from build123d import *

# Parameters (mm, degrees)
SKETCH1_W           = 3.81
SKETCH1_H           = 13.335
SKETCH1_R           = 1.1049
BOSS_EXTRUDE1_DEPTH = 9.525
SKETCH2_W           = 2.54
SKETCH2_H           = 13.335
BOSS_EXTRUDE2_DEPTH = 9.525


with BuildPart() as part:
    # Sketch1 → Boss-Extrude1 (new body)
    with BuildSketch(Plane(origin=(0, 0, 0), x_dir=(1, 0, 0), z_dir=(0, 1, 0))):
        Rectangle(SKETCH1_W, SKETCH1_H)
        with Locations(Location((0, 5.08, 0), (0, 0, 90))):
            Circle(SKETCH1_R, mode=Mode.SUBTRACT)
        with Locations(Location((0, -5.08, 0), (0, 0, 90))):
            Circle(SKETCH1_R, mode=Mode.SUBTRACT)
    extrude(amount=BOSS_EXTRUDE1_DEPTH)

    # Sketch2 → Boss-Extrude2 (add)
    with BuildSketch(Plane(origin=(0, 9.525, 0), x_dir=(1, 0, 0), z_dir=(0, 1, 0))):
        with Locations((-3.175, 0)):
            Rectangle(SKETCH2_W, SKETCH2_H)
    extrude(amount=-BOSS_EXTRUDE2_DEPTH)


solid = part.part
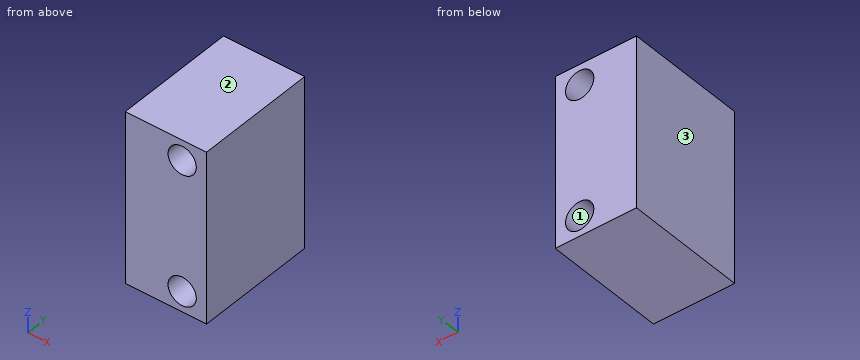
Model file for the job. Use its own axes, mm. Face numbers are marked on the shaded views. Coordinates: 2 decimals unless noted, no trailing zeros. Write each loop counter-clockwise with the first axis right and the second up, starting at its lowest first coordinate (ties: lowest second). Pieces come first, ordered by that corner, then holes. Notation, with made-up numbers: (77, 79) -> (134, 79) arc R14 ccw to (134, 92) -> close; hole circle Ø8 at (52.5, 11). An arc over 180 degrees is marked (long way). One line per item, written item: value. Start each with the question number.
1) Slice it at A-A on x = 0. Write the cut outline in (y, z) (1 decimal).
2) Pull direction Z, two halves, no side cores. Call the marked faces 1, 2 and 3: +Z half, -Z half, draft (parallel to the pull), parting line (faces both ways), or undercut.
3) Slice it at B-B on z = -5.08. Write the cut outline in (x, y) (3 decimals).
4) Probe probe 1 along Z at (x, y) = (-1, 4); probe 2 along Z at (x, y) = (0.5, 3.5); probe 3 along X at (y, z) = (7.25, 5.08) (3 decimals). List the from-to ranges inside material, lowest first.
5) Slice it at C-C on y = 2. Write the cut outline in (x, z) (1 decimal).
Answers follow:
1. outline: (0, -6.7) -> (9.5, -6.7) -> (9.5, -6.2) -> (0, -6.2) -> close; (0, -4) -> (9.5, -4) -> (9.5, 4) -> (0, 4) -> close; (0, 6.2) -> (9.5, 6.2) -> (9.5, 6.7) -> (0, 6.7) -> close
2. face 1: undercut
2. face 2: +Z half
2. face 3: draft
3. outline: (-4.445, 0) -> (-1.105, 0) -> (-1.105, 9.525) -> (-4.445, 9.525) -> close; (1.105, 0) -> (1.905, 0) -> (1.905, 9.525) -> (1.105, 9.525) -> close
4. probe 1: -6.67 to -5.55, -4.61 to 4.61, 5.55 to 6.67
4. probe 2: -6.67 to -6.07, -4.09 to 4.09, 6.07 to 6.67
4. probe 3: -4.445 to -1.105, 1.105 to 1.905
5. outline: (-4.4, -6.7) -> (1.9, -6.7) -> (1.9, 6.7) -> (-4.4, 6.7) -> close; hole circle Ø2.2 at (0, -5.1); hole circle Ø2.2 at (0, 5.1)
